from build123d import *

# Parameters (mm, degrees)
SCHIZZO1_W                   = 10
SCHIZZO1_H                   = 5.3
ESTRUSIONE_ESTRUSIONE1_DEPTH = 5.3
SCHIZZO2_R                   = 1.625
TAGLIO_ESTRUSIONE3_DEPTH     = 8.753225135
SCHIZZO3_W                   = 2.7
SCHIZZO3_H                   = 5.3
ESTRUSIONE_ESTRUSIONE2_DEPTH = 5.75
SCHIZZO4_R                   = 1.625
TAGLIO_ESTRUSIONE4_DEPTH     = 15.094325099
RACCORDO2_R                  = 2.65
RACCORDO3_R                  = 2.65


with BuildPart() as part:
    # Schizzo1 → Estrusione-Estrusione1 (new body)
    with BuildSketch(Plane.XY):
        Rectangle(SCHIZZO1_W, SCHIZZO1_H)
    extrude(amount=ESTRUSIONE_ESTRUSIONE1_DEPTH)

    # Schizzo2 → Taglio-Estrusione3 (cut, through all)
    with BuildSketch(Plane(origin=(0, 0, 0), x_dir=(-1, 0, 0), z_dir=(0, 0, -1))):
        Circle(SCHIZZO2_R)
    extrude(amount=-TAGLIO_ESTRUSIONE3_DEPTH, mode=Mode.SUBTRACT)

    # Schizzo3 → Estrusione-Estrusione2 (add)
    with BuildSketch(Plane(origin=(0, 2.65, 0), x_dir=(1, 0, 0), z_dir=(0, 1, 0))):
        with Locations((3.65, -2.65)):
            Rectangle(SCHIZZO3_W, SCHIZZO3_H)
        with Locations((-3.65, -2.65)):
            Rectangle(SCHIZZO3_W, SCHIZZO3_H)
    extrude(amount=ESTRUSIONE_ESTRUSIONE2_DEPTH)

    # Schizzo4 → Taglio-Estrusione4 (cut, through all)
    with BuildSketch(Plane.ZY.offset(5)):
        with Locations((2.684358211, 5.75)):
            Circle(SCHIZZO4_R)
    extrude(amount=-TAGLIO_ESTRUSIONE4_DEPTH, mode=Mode.SUBTRACT)

    # Raccordo2
    raccordo2_edges = [part.edges().sort_by_distance(p)[0] for p in [
        (3.65, 8.4, 0),
        (3.65, 8.4, 5.3),
        (-3.65, 8.4, 5.3),
        (-3.65, 8.4, 0),
    ]]
    fillet(raccordo2_edges, radius=RACCORDO2_R - 0.0001)  # a hair under: the kernel refuses the full size

    # Raccordo3
    raccordo3_edges = [part.edges().sort_by_distance(p)[0] for p in [
        (-5, -2.65, 2.65),
        (5, -2.65, 2.65),
    ]]
    fillet(raccordo3_edges, radius=RACCORDO3_R)


solid = part.part
Could you check a few things on this model? Use its own coordinates, in mm. A direction names the side the tool comes from. Give positions to 0.01 mm unless a question says otherwise; leave off trailing zeros. Write each loop counter-clockwise with the first axis right and the second up, starting at its lowest first coordinate (ties: lowest second). Pieces come first, ordered by that corner, then holes. Notation, with made-up numbers: (69.25, 27) -> (109.25, 27) arc R32 cw to (109.25, 57) -> close; hole circle Ø9 at (88.5, -23.75). An arc over 180 degrees is marked (long way). Answer as a JSON object with one key per item and string values.
Q1. Suppose I cut it at B-B on z = 3.05. Write out the boundary of the cut face in (x, y) (3 decimals), then the cut area to 3 significant figures.
Taken from the geometry:
{"outline": "(-5, 0) arc R2.65 ccw to (-2.35, -2.65) -> (2.35, -2.65) arc R2.65 ccw to (5, 0) -> (5, 4.167) -> (2.3, 4.167) -> (2.3, 2.65) -> (-2.3, 2.65) -> (-2.3, 4.167) -> (-5, 4.167) -> close; (-5, 7.333) -> (-2.3, 7.333) -> (-2.3, 8.37) -> (-5, 8.37) -> close; (2.3, 7.333) -> (5, 7.333) -> (5, 8.37) -> (2.3, 8.37) -> close; hole circle Ø3.25 at (0, 0)", "area": "55.5 mm²"}
Q2. Suppose I cut it at C-C on y = 3.5. Write out the boundary of the cut face in (x, z).
Taken from the geometry:
{"outline": "(-5, 0) -> (-2.3, 0) -> (-2.3, 5.3) -> (-5, 5.3) -> close; (2.3, 0) -> (5, 0) -> (5, 5.3) -> (2.3, 5.3) -> close"}
Q3. Suppose I cut it at A-A on x = 0. Write out the boundary of the cut face in (y, z) (3 decimals), then the cut area to 3 significant figures.
Taken from the geometry:
{"outline": "(-2.65, 0) -> (-1.625, 0) -> (-1.625, 5.3) -> (-2.65, 5.3) -> close; (1.625, 0) -> (2.65, 0) -> (2.65, 5.3) -> (1.625, 5.3) -> close", "area": "10.9 mm²"}
Q4. We'd pull the mould along Z, two halves only. Please class faces 3 (the cylindrical face through (-3.67, 6.85, 1.49)), 4 (the flat face through (5, 3, 3)), 5 (the cylindrical face through (3.669, 7.603, 4.544)): released by +Z, released by -Z, zero draft, split by the parting line, or undercut.
Taken from the geometry:
{"face 3": "undercut", "face 4": "zero draft", "face 5": "released by +Z"}
Q5. Which directions (+Z, -Z, +X, -X, +Y, -Y) give clear straight access to the entire face, cutting with the end or side of a thin tool? Please do faces 1 (the flat face through (0, 2.65, 3)), 2 (the cylindrical face through (-3.631, 7.603, 0.756)).
Taken from the geometry:
{"face 1": "+Z, -Z, +Y", "face 2": "-Z, +X, -X, +Y"}
Q6. Please list where these lines run through material, in increasing order: L1, parallel to X at y = 4, z = 3.8; L2, parallel to Y at x = 0, z = 2.45 (3 decimals); L3, parallel to Z at x = 3, y = 6.75.
Taken from the geometry:
{"L1": "x = -5 to -2.3, 2.3 to 5", "L2": "y = -2.65 to -1.625, 1.625 to 2.65", "L3": "z = 0.2 to 1.4, 3.97 to 5.1"}
